The listing builds one solid part. Answer for the finished solid, in the listing's coordinates (mm). A direction names the side the tool comes from. Give positions to 0.01 mm unless a question says otherwise; leave off trailing zeros. Write each loop counter-clockwise with the first axis right and the second up, starting at its lowest first coordinate (ties: lowest second). Pieces come first, ordered by that corner, then holes. Notation, with made-up numbers: (68, 51) - (121, 51) arc R7 cw to (121, 56) - close; hole circle Ø2 at (58.5, -4). An arc over 180 degrees is marked (long way). One line per item, written item: value. Start each with the question number.
from build123d import *

# Parameters (mm, degrees)
SKETCH1_W           = 18.542
SKETCH1_H           = 17.78
BOSS_EXTRUDE4_DEPTH = 1.905
SKETCH4_W           = 18.542
SKETCH4_H           = 17.78
BOSS_EXTRUDE5_DEPTH = 1.905
BOSS_EXTRUDE6_DEPTH = 18.542
SKETCH7_W           = 8.89
SKETCH7_H           = 10.16
BOSS_EXTRUDE7_DEPTH = 1.905
SKETCH8_W           = 8.89
SKETCH8_H           = 10.16
BOSS_EXTRUDE8_DEPTH = 1.905
SKETCH9_W           = 6.35
SKETCH9_H           = 5.08
BOSS_EXTRUDE9_DEPTH = 2.54
SKETCH10_W          = 1.27
SKETCH10_H          = 5.08
CUT_EXTRUDE1_DEPTH  = 23.269948832


with BuildPart() as part:
    # Sketch1 → Boss-Extrude4 (new body)
    with BuildSketch(Plane.XY):
        Rectangle(SKETCH1_W, SKETCH1_H)
    extrude(amount=-BOSS_EXTRUDE4_DEPTH)



with BuildPart() as body_2:
    # Sketch4 → Boss-Extrude5 (new body)
    with BuildSketch(Plane.XY.offset(-12.7)):
        Rectangle(SKETCH4_W, SKETCH4_H)
    extrude(amount=BOSS_EXTRUDE5_DEPTH)


with BuildPart() as part_1:
    add(part.part)

    add(body_2.part)  # Boss-Extrude6 merges body 2
    # Sketch6 → Boss-Extrude6 (add)
    with BuildSketch(Plane.ZY.offset(9.271)):
        with BuildLine():
            Line((-12.7, 8.89), (-10.795, 8.89))
            ThreePointArc((-10.795, 8.89), (-6.35, 13.335), (-1.905, 8.89))
            Line((-1.905, 8.89), (0, 8.89))
            ThreePointArc((0, 8.89), (-6.35, 15.24), (-12.7, 8.89))
        make_face()
    extrude(amount=-BOSS_EXTRUDE6_DEPTH)

    # Sketch7 → Boss-Extrude7 (add)
    with BuildSketch(Plane.ZY.offset(9.271)):
        with Locations((-6.35, -3.81)):
            Rectangle(SKETCH7_W, SKETCH7_H)
    extrude(amount=-BOSS_EXTRUDE7_DEPTH)

    # Sketch8 → Boss-Extrude8 (add)
    with BuildSketch(Plane(origin=(9.271, 0, 0), x_dir=(0, 0, -1), z_dir=(1, 0, 0))):
        with Locations((6.35, -3.81)):
            Rectangle(SKETCH8_W, SKETCH8_H)
    extrude(amount=-BOSS_EXTRUDE8_DEPTH)

    # Sketch9 → Boss-Extrude9 (add)
    with BuildSketch(Plane(origin=(9.271, 0, 0), x_dir=(0, 0, -1), z_dir=(1, 0, 0))):
        with Locations((6.35, -1.27)):
            Rectangle(SKETCH9_W, SKETCH9_H)
    extrude(amount=BOSS_EXTRUDE9_DEPTH)

    # Sketch10 → Cut-Extrude1 (cut, through all)
    with BuildSketch(Plane(origin=(0, 1.27, 0), x_dir=(1, 0, 0), z_dir=(0, 1, 0))):
        with Locations((9.906, 6.35)):
            Rectangle(SKETCH10_W, SKETCH10_H)
    extrude(amount=-CUT_EXTRUDE1_DEPTH, mode=Mode.SUBTRACT)


solid = part_1.part
Item 1: For faces 4 (the flat face through (-8, 1.27, -6)), 5 (the flat face through (11, -1, -3.175)), 6 (the flat face through (10.541, -1, -6)), 7 (the flat face through (7.366, -4, -6)), determine the directions among +Z, -Z, +X, -X, +Y, -Y from which every point of the face is accessible in a straight line to the end or side of a thin tool.
Item 2: Find section D-D on y = -7.5. Determine the outline of the cut face in (x, z) (3 decimals), plus the area to 3 significant figures.
Item 3: Find section C-C on y = -0.5. Determine the outline of the cut face in (x, z) (3 decimals), plus the area to 3 significant figures.
Item 4: Find section A-A on z = -6.35. Determine the outline of the cut face in (x, y) (3 decimals), plus the area to 3 significant figures.
Item 5: Each of these flat-tipped pins is pushed along its axis until it touches: pin 1 Ø0.8 at (x, y) = (10.5, 0) entering from +Z (3 decimals); pin 2 Ø3 at (x, y) = (11, 0) entering from -Z (3 decimals); pin 3 Ø2.5 at (y, z) = (-6.5, -4.5) entering from +X. Where does it stop, or does it pass through?
Item 6: The mould has two halves that part along Z. Classify faces 1 (the flat face through (0, 0, 0)), 2 (the flat face through (11, -1, -9.525)), 3 (the flat face through (0, 0, -1.905)): +Z half, -Z half, draft (parallel to the pull), parting line (faces both ways), or undercut.
Item 7: Find section B-B on y = 6. Determine the outline of the cut face in (x, z) (3 decimals), plus the area to 3 significant figures.
Item 8: Straight lines are drawn through the part: line 1 along X through (y, z) = (-0.75, -7.75); line 2 along Z through (x, y) = (-7.25, 2) (3 decimals); line 3 along X through (y, z) = (-4.5, -8.5). For each, find the intervals that lie inside material, in ascending order.
Values:
1. face 4: +X, -X
1. face 5: +Z, +X, +Y, -Y
1. face 6: +Y, -Y
1. face 7: -Y
2. outline: (-9.271, -12.7) - (9.271, -12.7) - (9.271, 0) - (-9.271, 0) - close; hole (-7.366, -10.795) - (7.366, -10.795) - (7.366, -1.905) - (-7.366, -1.905) - close
2. area: 105 mm^2
3. outline: (-9.271, -12.7) - (9.271, -12.7) - (9.271, -9.525) - (11.811, -9.525) - (11.811, -3.175) - (9.271, -3.175) - (9.271, 0) - (-9.271, 0) - close; hole (-7.366, -10.795) - (7.366, -10.795) - (7.366, -1.905) - (-7.366, -1.905) - close; hole (9.271, -8.89) - (10.541, -8.89) - (10.541, -3.81) - (9.271, -3.81) - close
3. area: 114 mm^2
4. outline: (-9.271, -8.89) - (-7.366, -8.89) - (-7.366, 1.27) - (-9.271, 1.27) - close; (-9.271, 13.335) - (9.271, 13.335) - (9.271, 15.24) - (-9.271, 15.24) - close; (7.366, -8.89) - (9.271, -8.89) - (9.271, 1.27) - (7.366, 1.27) - close; (10.541, -3.81) - (11.811, -3.81) - (11.811, 1.27) - (10.541, 1.27) - close
4. area: 80.5 mm^2
5. pin 1: z = -3.175
5. pin 2: z = -9.525
5. pin 3: x = 9.27
6. face 1: +Z half
6. face 2: -Z half
6. face 3: undercut
7. outline: (-9.271, -12.7) - (9.271, -12.7) - (9.271, -10.795) - (-9.271, -10.795) - close; (-9.271, -1.905) - (9.271, -1.905) - (9.271, 0) - (-9.271, 0) - close
7. area: 70.6 mm^2
8. line 1: -9.27 to -7.37, 7.37 to 9.27, 10.54 to 11.81
8. line 2: -12.7 to -10.795, -1.905 to 0
8. line 3: -9.27 to -7.37, 7.37 to 9.27
